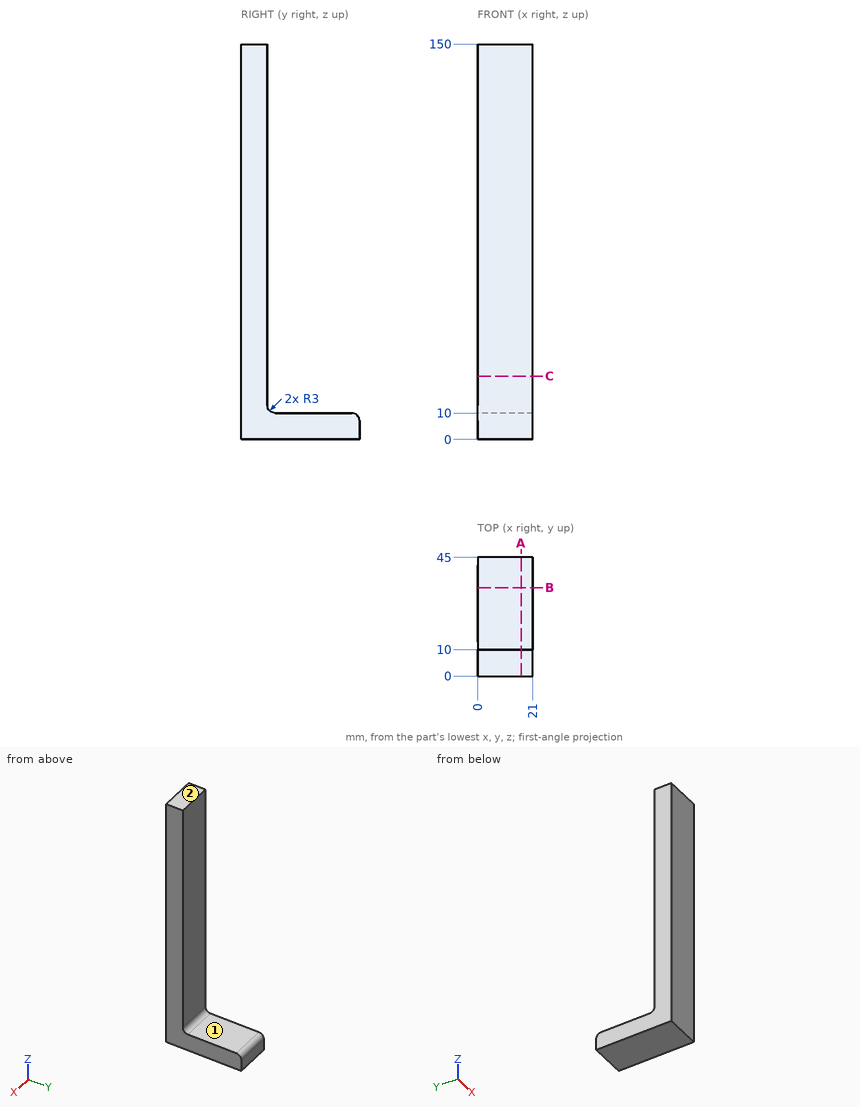
Drawing for the job (mm, zero at the part's lowest x, y, z). A direction names the side the tool comes from. Coordinates: 2 decimals unless noted, no trailing zeros. Loops run counter-clockwise (first coordinate to the right, second up) from the corner with the lowest first, then second, coordinate; pieces in that order, holes last. Notation, with made-up numbers: (78.5, 53) - (99.5, 53) arc R30 cw to (99.5, 83) - close; hole circle Ø11 at (80.5, 87.25). An arc over 180 degrees is marked (long way). Return JSON: item names as keys, results as strings.
1. Probe L1, parallel to Y at x = 6, z = 101; L2, parallel to Z at x = 5.5, y = 43. List the from-to ranges inside material, lowest first. Write a range as from..to.
Result:
{"L1": "y = 0..10", "L2": "z = 0..9.83"}
2. Drop flat-ended pins along their axis: pin 1 (1 mm diameter, centred on x = 3, y = 39.5, fed in from +Z); pin 2 (8 mm diameter, centred on x = 12, y = 15.5, fed in from +Z); pin 3 (12 mm diameter, centred on x = 2, z = 78, fed in from +Y). Give the stop position or say it passes through.
Result:
{"pin 1": "stops at z = 10", "pin 2": "stops at z = 10.4", "pin 3": "stops at y = 10"}
3. Band-saw the part on B-B (y = 33.5). Give the cut face in (x, z), and give its area (3 significant figures).
Result:
{"outline": "(0, 0) - (21, 0) - (21, 10) - (0, 10) - close", "area": "210 mm2"}
4. 3-axis set-ups, long thin cutter, end or side, ignore diameter. For the marked faces 1 and 2: which of +Z, -Z, +X, -X, +Y, -Y reach the whole face in a straight line?
Result:
{"face 1": "+Z, +X, -X, +Y", "face 2": "+Z, +X, -X, +Y, -Y"}
5. Band-saw the part on A-A (x = 16.5). Give the cut face in (y, z), and give its area (3 significant figures).
Result:
{"outline": "(0, 0) - (45, 0) - (45, 7) arc R3 ccw to (42, 10) - (13, 10) arc R3 cw to (10, 13) - (10, 150) - (0, 150) - close", "area": "1,850 mm2"}
